```python
from build123d import *

# Parameters (mm, degrees)
BOSS_EXTRUDE1_DEPTH = 8
SKETCH2_R           = 2.75
CUT_EXTRUDE1_DEPTH  = 9
SKETCH3_R           = 5
CUT_EXTRUDE2_DEPTH  = 4.2


with BuildPart() as part:
    # Sketch1 → Boss-Extrude1 (new body)
    with BuildSketch(Plane(origin=(0, 0, 0), x_dir=(1, 0, 0), z_dir=(0, 1, 0))):
        Polygon((7.5, 25), (6.5, 25), (6.5, -25), (7.5, -25), (7.5, -35), (-7.5, -35), (-7.5, 35), (7.5, 35), align=None)
    extrude(amount=BOSS_EXTRUDE1_DEPTH)

    # Sketch2 → Cut-Extrude1 (cut, through all)
    with BuildSketch(Plane(origin=(0, 8, 0), x_dir=(1, 0, 0), z_dir=(0, 1, 0))):
        with Locations((-0.5, 17.5)):
            Circle(SKETCH2_R)
        with Locations((-0.5, -17.5)):
            Circle(SKETCH2_R)
    extrude(amount=-CUT_EXTRUDE1_DEPTH, mode=Mode.SUBTRACT)

    # Sketch3 → Cut-Extrude2 (cut)
    with BuildSketch(Plane(origin=(0, 8, 0), x_dir=(1, 0, 0), z_dir=(0, 1, 0))):
        with Locations((-0.5, 17.5)):
            Circle(SKETCH3_R)
        with Locations((-0.5, -17.5)):
            Circle(SKETCH3_R)
    extrude(amount=-CUT_EXTRUDE2_DEPTH, mode=Mode.SUBTRACT)


solid = part.part
```
Verification items for the finished model (mm, model axes). A direction names the side the tool comes from. Coordinates: 2 decimals unless noted, no trailing zeros. Loops run counter-clockwise (first coordinate to the right, second up) from the corner with the lowest first, then second, coordinate; pieces in that order, holes last. Notation, with made-up numbers: (9, 21) - (53, 21) arc R22 ccw to (53, 41) - close; hole circle Ø3 at (-7.5, -6.75). An arc over 180 degrees is marked (long way). Put each result on its own line as item: value.
Item 1: Gauge pin test, flat end, axial feed: pin 1 Ø7 at (x, z) = (-0.5, -17.5) entering from +Y. Record the tip position at first contact, or that the pin passes through.
Conclusion:
pin 1: stops at y = 3.8
Item 2: Section check A-A (x = -0.5). Enter the section's corners in (y, z).
Conclusion:
outline: (0, -35) - (8, -35) - (8, -22.5) - (3.8, -22.5) - (3.8, -20.25) - (0, -20.25) - close; (0, -14.75) - (3.8, -14.75) - (3.8, -12.5) - (8, -12.5) - (8, 12.5) - (3.8, 12.5) - (3.8, 14.75) - (0, 14.75) - close; (0, 20.25) - (3.8, 20.25) - (3.8, 22.5) - (8, 22.5) - (8, 35) - (0, 35) - close
Item 3: Section check C-C (z = 17.5). Enter the section's corners in (x, y), then the cut area to 3 significant figures.
Conclusion:
outline: (-7.5, 0) - (-3.25, 0) - (-3.25, 3.8) - (-5.5, 3.8) - (-5.5, 8) - (-7.5, 8) - close; (2.25, 0) - (6.5, 0) - (6.5, 8) - (4.5, 8) - (4.5, 3.8) - (2.25, 3.8) - close
area: 49.1 mm2
Item 4: Set-up check for faces 1 (the face through (6.5, 4, 0)), 2 (the face through (0, 0, 0)), 3 (the face through (2, 3.8, -15)): record each of +Z, -Z, +X, -X, +Y, -Y from which the full face is reachable in a straight line by a thin tool's end or side.
Conclusion:
face 1: +X, +Y, -Y
face 2: +Z, -Z, +X, -X, -Y
face 3: +Y
Item 5: Section check B-B (y = 1.75). Enter the section's corners in (x, z), then the cut area to 3 significant figures.
Conclusion:
outline: (-7.5, -35) - (7.5, -35) - (7.5, -25) - (6.5, -25) - (6.5, 25) - (7.5, 25) - (7.5, 35) - (-7.5, 35) - close; hole circle Ø5.5 at (-0.5, -17.5); hole circle Ø5.5 at (-0.5, 17.5)
area: 952 mm2
Item 6: Scan lines: line 1 along Z through (x, y) = (-0.5, 6.65); line 2 along Z through (x, y) = (-0.5, 1.25); line 3 along X through (y, z) = (5.25, -17.5). Record each from-to range of solid material in increasing order.
Conclusion:
line 1: z = -35 to -22.5, -12.5 to 12.5, 22.5 to 35
line 2: z = -35 to -20.25, -14.75 to 14.75, 20.25 to 35
line 3: x = -7.5 to -5.5, 4.5 to 6.5
Item 7: Section check D-D (z = 3.5). Enter the section's corners in (x, y).
Conclusion:
outline: (-7.5, 0) - (6.5, 0) - (6.5, 8) - (-7.5, 8) - close
Item 8: Draft check along Z on faces 4 (the face through (0, 8, 0)), 5 (the face through (0, 4, 35)), 6 (the face through (2, 3.8, 20)). Enter one of: pulls with the +Z half, pulls with the -Z half, needs draft (parallel to the pull), parting line crosses it, or undercut.
Conclusion:
face 4: needs draft
face 5: pulls with the +Z half
face 6: undercut
